Source: CAD feature listing. Evaluate the final solid. Frame: model axes, mm. A direction names the side the tool comes from. Round coordinates to 2 decimals unless told otherwise and drop trailing zeros. Loops run counter-clockwise (first coordinate to the right, second up) from the corner with the lowest first, then second, coordinate; pieces in that order, holes last.
Item 1: Access query for faces 1 (the flat face through (-7, 0, 13)), 2 (the flat face through (1, 0, 2)), 3 (the flat face through (-5, 6.5, 14)). Directions: +Z, -Z, +X, -X, +Y, -Y. A direction counts if a zero-diameter tool reaches every point of the face in a straight line with its end or side. Return the directions, or none.
Item 2: Ray query, L1, parallel to Y at x = -16, z = 27.4; L2, parallel to Z at x = -7.5, y = 5.5; L3, parallel to X at y = 4, z = 23.5. Return the intervals inside material, ascending.
Item 3: Section query D-D on x = -16. Return loops of the section in (y, z), then the cut area to 3 significant figures.
Item 4: Section query C-C on y = -3.5. Return loops of the section in (x, z), then the cut area to 3 significant figures.
Item 5: Section query A-A on y = 0. Return loops of the section in (x, z), then the cut area to 3 significant figures.
Item 6: Pull-direction query (X, two-part tool) for faces 4 (the cylindrical face through (-17.5, 0.07, 26.99)), 5 (the flat face through (-14, 0, 26)), 6 (the cylindrical face through (5.796, 0.676, 0.986)), 7 (the flat face through (-1, 0, 15)); classes: released by +X, released by -X, zero draft, split by the parting line, or undercut.
Item 7: First-contact query: P1, Ø4, axis at x = -16, y = 0, coming from the -Z side; P2, Ø2, axis at y = 3, z = 10.5, coming from the -X side; P3, Ø6.5, axis at x = 2.5, y = 0, coming from the +Z side. Flat tips, straight axial feed; report the tip coordinate or a pass-through.
Item 8: Section query B-B on x = 3.65. Return loops of the section in (y, z), then the cut area to 3 significant figures.
```python
from build123d import *

# Parameters (mm, degrees)
SZKIC1_W                    = 14
SZKIC1_H                    = 13
SZKIC1_R                    = 2.25
DODANIE_WYCI_GNI_CIE1_DEPTH = 2
SZKIC2_W                    = 6
SZKIC2_H                    = 13
DODANIE_WYCI_GNI_CIE2_DEPTH = 24
SZKIC3_W                    = 20
SZKIC3_H                    = 13
SZKIC3_R                    = 1.5
DODANIE_WYCI_GNI_CIE3_DEPTH = 2


with BuildPart() as part:
    # Szkic1 → Dodanie-wyciągnięcie1 (new body)
    with BuildSketch(Plane.XY):
        Rectangle(SZKIC1_W, SZKIC1_H)
        with Locations((3.65, 0)):
            Circle(SZKIC1_R, mode=Mode.SUBTRACT)
    extrude(amount=DODANIE_WYCI_GNI_CIE1_DEPTH)

    # Szkic2 → Dodanie-wyciągnięcie2 (add)
    with BuildSketch(Plane.XY.offset(2)):
        with Locations((-4, 0)):
            Rectangle(SZKIC2_W, SZKIC2_H)
    extrude(amount=DODANIE_WYCI_GNI_CIE2_DEPTH)

    # Szkic3 → Dodanie-wyciągnięcie3 (add)
    with BuildSketch(Plane.XY.offset(26)):
        with Locations((-11, 0)):
            Rectangle(SZKIC3_W, SZKIC3_H)
        with Locations((-16, 0)):
            Circle(SZKIC3_R, mode=Mode.SUBTRACT)
    extrude(amount=DODANIE_WYCI_GNI_CIE3_DEPTH)


solid = part.part
```
Data:
1. face 1: -Z, -X, +Y, -Y
1. face 2: +Z, +X, +Y, -Y
1. face 3: +Z, -Z, +X, -X, +Y
2. L1: y = -6.5 to -1.5, 1.5 to 6.5
2. L2: z = 26 to 28
2. L3: x = -7 to -1
3. outline: (-6.5, 26) - (-1.5, 26) - (-1.5, 28) - (-6.5, 28) - close; (1.5, 26) - (6.5, 26) - (6.5, 28) - (1.5, 28) - close
3. area: 20.0 mm2
4. outline: (-21, 26) - (-7, 26) - (-7, 0) - (7, 0) - (7, 2) - (-1, 2) - (-1, 28) - (-21, 28) - close
4. area: 212 mm2
5. outline: (-21, 26) - (-17.5, 26) - (-17.5, 28) - (-21, 28) - close; (-14.5, 26) - (-7, 26) - (-7, 0) - (1.4, 0) - (1.4, 2) - (-1, 2) - (-1, 28) - (-14.5, 28) - close; (5.9, 0) - (7, 0) - (7, 2) - (5.9, 2) - close
5. area: 197 mm2
6. face 4: undercut
6. face 5: zero draft
6. face 6: undercut
6. face 7: released by +X
7. P1: stops at z = 26
7. P2: stops at x = -7
7. P3: stops at z = 2
8. outline: (-6.5, 0) - (-2.25, 0) - (-2.25, 2) - (-6.5, 2) - close; (2.25, 0) - (6.5, 0) - (6.5, 2) - (2.25, 2) - close
8. area: 17.0 mm2
